from build123d import *

# Parameters (mm, degrees)
CROQUIS1_R              = 15
SALIENTE_EXTRUIR1_DEPTH = 20
CROQUIS2_R              = 15
SALIENTE_EXTRUIR2_DEPTH = 12
SALIENTE_EXTRUIR3_DEPTH = 6


with BuildPart() as part:
    # Croquis1 → Saliente-Extruir1 (new body)
    with BuildSketch(Plane.XY):
        with BuildLine():
            Line((-50, 0), (50, 0))
            ThreePointArc((50, 0), (37.97918472, 4.97918472), (33, 17))
            Line((33, 17), (33, 100))
            ThreePointArc((33, 100), (0, 133), (-33, 100))
            Line((-33, 100), (-33, 17))
            ThreePointArc((-33, 17), (-37.97918472, 4.97918472), (-50, 0))
        make_face()
        with Locations((0, 100)):
            Circle(CROQUIS1_R, mode=Mode.SUBTRACT)
    extrude(amount=-SALIENTE_EXTRUIR1_DEPTH)

    # Croquis2 → Saliente-Extruir2 (add)
    with BuildSketch(Plane(origin=(0, 0, 0), x_dir=(1, 0, 0), z_dir=(0, 1, 0))):
        with BuildLine():
            Line((-50, 20), (-50, -91))
            ThreePointArc((-50, -91), (-45.899494937, -100.899494937), (-36, -105))
            Line((-36, -105), (36, -105))
            ThreePointArc((36, -105), (45.899494937, -100.899494937), (50, -91))
            Line((50, -91), (50, 20))
            Line((50, 20), (-50, 20))
        make_face()
        with Locations((0, -80)):
            Circle(CROQUIS2_R, mode=Mode.SUBTRACT)
    extrude(amount=-SALIENTE_EXTRUIR2_DEPTH)

    # Croquis3 → Saliente-Extruir3 (add, symmetric)
    with BuildSketch(Plane(origin=(0, 0, 0), x_dir=(0, 0, -1), z_dir=(1, 0, 0))):
        Polygon((0, 50), (-50, 0), (0, 0), align=None)
    extrude(amount=SALIENTE_EXTRUIR3_DEPTH, both=True)

    # Croquis5 → Revolución1 (revolve)
    with BuildSketch(Plane(origin=(0, 0, 0), x_dir=(0, 0, -1), z_dir=(1, 0, 0))):
        Polygon((20, 126), (60, 119), (60, 110), (20, 110), align=None)
    revolve(axis=Axis((0, 100, 0), (0, 0, -1)))

    # Croquis6 → Revolución2 (revolve)
    with BuildSketch(Plane(origin=(0, 0, 0), x_dir=(0, 0, -1), z_dir=(1, 0, 0))):
        Polygon((-105, -12), (-95, -62), (-88, -62), (-88, -12), align=None)
    revolve(axis=Axis((0, -12, 80), (0, -1, 0)))


solid = part.part
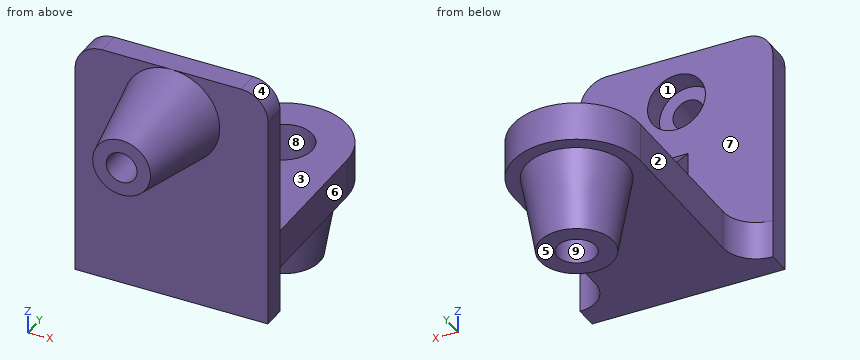
Here's how the part is built. I have some questions about the finished solid (model axes, mm). Face numbers are marked on the shaded views. A direction names the side the tool comes from. Round coordinates to 2 decimals unless told otherwise and drop trailing zeros. Write each loop counter-clockwise with the first axis right and the second up, starting at its lowest first coordinate (ties: lowest second). Pieces come first, ordered by that corner, then holes. Notation, with made-up numbers: (-38, -13.75) -> (5, -13.75) arc R22 cw to (5, 13.25) -> close; hole circle Ø6 at (22, 25). An arc over 180 degrees is marked (long way). One line per item, written item: value.
1) Suppose I cut it at B-B on y = -7. List the corners of the cut face in (x, z) for me.
Filled sheet:
outline: (-50, -20) -> (50, -20) -> (50, 91) arc R14 ccw to (36, 105) -> (-36, 105) arc R14 ccw to (-50, 91) -> close; hole circle Ø30 at (0, 80)
2) Suppose I cut it at D-D on y = 21. List the corners of the cut face in (x, z) for me, plus the area to 3 significant figures.
Filled sheet:
outline: (-33, -20) -> (33, -20) -> (33, 0) -> (6, 0) -> (6, 29) -> (-6, 29) -> (-6, 0) -> (-33, 0) -> close
area: 1,670 mm2
3) For the marked faces 1, 2, 3, 4 and 5, which set-ups out of +Z, -Z, +X, -X, +Y, -Y let a thin tool reach every point of the face, with its end or its side?
Filled sheet:
face 1: +Y
face 2: +Z, -Z, -X, +Y
face 3: +Z, +Y
face 4: +Z, +X, +Y, -Y
face 5: -Z, +X, -X, +Y, -Y
4) If I drill on line 1 (Y direction, x = 4.5, z = 93.5); line 2 (Y direction, x = 20, z = 43.5); line 3 (Z direction, x = 14, y = 30), over which ranges is the centre line in solid material (lowest first)? Write a range as [from, to].
Filled sheet:
line 1: y = [-62, -12]
line 2: y = [-12, 0]
line 3: z = [-20, 0]
5) Suppose I cut it at A-A on z = 80. List the corners of the cut face in (x, y) for me, plus the area to 3 significant figures.
Filled sheet:
outline: (-50, -12) -> (-25, -12) -> (-15, -62) -> (-8, -62) -> (-8, -12) -> (-15, -12) -> (-15, 0) -> (-50, 0) -> close; (8, -62) -> (15, -62) -> (25, -12) -> (50, -12) -> (50, 0) -> (15, 0) -> (15, -12) -> (8, -12) -> close
area: 2,040 mm2
6) I'm going to push flat-ended pins straight in: pin 1 Ø5 at (x, y) = (31.5, 51) entering from -Z; pin 2 Ø25 at (y, z) = (32.5, 30.5) entering from +X; pin 3 Ø10 at (x, z) = (18.5, 11.5) entering from +Y; pin 4 Ø12 at (x, y) = (0, 100) entering from +Z. Where does each tip first touch, or does it pass through?
Filled sheet:
pin 1: stops at z = -20
pin 2: stops at x = 6
pin 3: stops at y = 0
pin 4: passes through
7) We'd pull the mould along X, two halves only. Please class the marked faces 6, 7, 8 and 9: released by +X, released by -X, zero draft, split by the parting line, or undercut.
Filled sheet:
face 6: released by +X
face 7: zero draft
face 8: undercut
face 9: undercut
8) Suppose I cut it at C-C on z = 35. List the corners of the cut face in (x, y) for me, plus the area to 3 significant figures.
Filled sheet:
outline: (-50, -12) -> (50, -12) -> (50, 0) -> (6, 0) -> (6, 15) -> (-6, 15) -> (-6, 0) -> (-50, 0) -> close
area: 1,380 mm2
